Autodesk Inventor part; units mm, degrees
ref_plane "YZ Plane" through (0, 0, 0) normal (1, 0, 0) x (0, 1, 0)
ref_plane "XZ Plane" through (0, 0, 0) normal (0, 1, 0) x (-1, 0, 0)
ref_plane "XY Plane" through (0, 0, 0) normal (0, 0, 1) x (1, 0, 0)
sketch "Sketch1" plane through (0, 0, 0) normal (0, 0, 1) x (1, 0, 0)
  arc A0 (1.5, 7.5) -> (-1.3846, 6.9231) centre (0, 7.5) ccw
  arc A1 (-1.3846, -6.9231) -> (1.5, -7.5) centre (0, -7.5) ccw
  arc A2 (-10.3524, -1.1528) -> (-10.356, 1.1198) centre (-12, -0.0191) ccw
  arc A3 (10.1342, 4.2777) -> (-10.6479, 2.7607) centre (0, 0) ccw
  arc A4 (-10.6391, -2.7946) -> (10.134, -4.278) centre (0, 0) ccw
  arc A5 (-10.6479, 2.7607) -> (-10.356, 1.1198) centre (-8.7119, 2.2588) ccw
  arc A6 (-10.3524, -1.1528) -> (-10.6391, -2.7946) centre (-8.7047, -2.2865) ccw
  arc A7 (-1, 5) -> (-1.3846, 6.9231) centre (-6, 5) ccw
  arc A8 (-1.3846, -6.9231) -> (-1, -5) centre (-6, -5) ccw
  line L0 (1.5, 7.5) -> (1.5, 6.5)
  line L1 (1.4995, -6.5) -> (1.4995, -7.5382)
  line L2 (6.4997, -1.5002) -> (8.2915, -1.5002)
  line L3 (6.4998, 1.5) -> (8.2915, 1.4999)
  arc A9 (6.4997, -1.5002) -> (1.4995, -6.5) centre (6.4995, -6.5002) ccw
  arc A10 (1.5, 6.5) -> (6.4998, 1.5) centre (6.5, 6.5) ccw
  arc A11 (10.134, -4.278) -> (8.2915, -1.5002) centre (8.2915, -3.5002) ccw
  arc A12 (8.2915, 1.4999) -> (10.1342, 4.2777) centre (8.2916, 3.4999) ccw
  line L4 (-6, 2) -> (-4, 2)
  line L5 (-4, -2) -> (-6, -2)
  line L6 (-7, -1) -> (-7, 1)
  arc A13 (-6, 2) -> (-7, 1) centre (-6, 1) ccw
  arc A14 (-7, -1) -> (-6, -2) centre (-6, -1) ccw
  line L7 (-1, -5) -> (-1, -5)
  line L8 (-1, 5) -> (-1, 5)
  arc A15 (-4, 2) -> (-1, 5) centre (-4, 5) ccw
  arc A16 (-1, -5) -> (-4, -2) centre (-4, -5) ccw
  point P0 (10.8972, -1.5003)
  point P1 (10.8973, 1.4999)
  point P2 (1.5, 1.5002)
  point P3 (1.4997, -1.5)
  point P4 (-1, -6.382)
  point P5 (-1, 6.382)
  point P6 (-7, 2)
  point P7 (-7, -2)
  point P8 (-4.7429, 0)
  dimension "d5" = 3
  dimension "d6" = 3
  dimension "d7" = 15
  dimension "d18" = 7.5
  dimension "d20" = 4
  dimension "d21" = 12
  dimension "d22" = 2
  dimension "d26" = 5
  dimension "d27" = 5
  dimension "d28" = 2
  dimension "d30" = 4
  dimension "d31" = 1
  dimension "d32" = 3
  dimension "d33" = 7
extrude "Extrusion2" add sketch "Sketch1" along normal blind 3
properties part number "020914 Aft Middle Endcap" material "Polycarbonate, Clear"
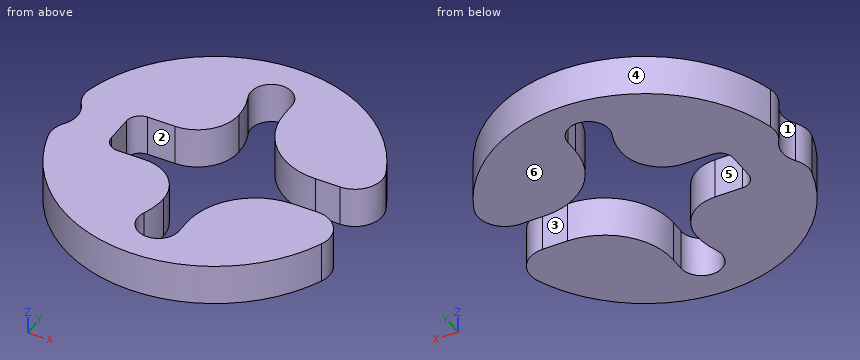
Design review of the part built by this model. Coordinates are the model's own, in mm. Face numbers are marked on the shaded views. A direction names the side the tool comes from. Round coordinates to 2 decimals unless told otherwise and drop trailing zeros. Write each loop counter-clockwise with the first axis right and the second up, starting at its lowest first coordinate (ties: lowest second). Pieces come first, ordered by that corner, then holes. Notation, with made-up numbers: (-30, -22.5) -> (17, -22.5) arc R10 cw to (17, -8.5) -> close; hole circle Ø3 at (-28.5, -38.5). An arc over 180 degrees is marked (long way). Answer in a Markdown table with one row per item.
Q1. Take a section at B-B, the plane y = -4.75. State the section outline as (x, z) points, then the cut area to 3 significant figures.
The answers:
| item | result |
|---|---|
| outline | (-9.92, 0) -> (-1.01, 0) -> (-1.01, 3) -> (-9.92, 3) -> close; (1.82, 0) -> (9.92, 0) -> (9.92, 3) -> (1.82, 3) -> close |
| area | 51.1 mm² |
Q2. Take a section at C-C, the plane z = 2.3. State the section outline as (x, y) points, then the cut area to 3 significant figures.
The answers:
| item | result |
|---|---|
| outline | (-10.65, 2.76) arc R2 ccw to (-10.36, 1.12) arc R2 cw to (-10.35, -1.15) arc R2 ccw to (-10.64, -2.79) arc R11 ccw to (10.13, -4.28) arc R2 ccw to (8.29, -1.5) -> (6.5, -1.5) arc R5 ccw to (1.5, -6.5) -> (1.5, -7.5) arc R1.5 cw (long way) to (-1.38, -6.92) arc R5 ccw to (-1, -5) arc R3 ccw to (-4, -2) -> (-6, -2) arc R1 cw to (-7, -1) -> (-7, 1) arc R1 cw to (-6, 2) -> (-4, 2) arc R3 ccw to (-1, 5) arc R5 ccw to (-1.38, 6.92) arc R1.5 cw (long way) to (1.5, 7.5) -> (1.5, 6.5) arc R5 ccw to (6.5, 1.5) -> (8.29, 1.5) arc R2 ccw to (10.13, 4.28) arc R11 ccw to start |
| area | 262 mm² |
Q3. For the marked faces 1, 2 and 3, list the 3-axis set-ups (+Z, -Z, +X, -X, +Y, -Y) from which the entire face can be reached by the end or side of a thin tool; tool diameter is ignored.
The answers:
| item | result |
|---|---|
| face 1 | +Z, -Z, -X |
| face 2 | +Z, -Z |
| face 3 | +Z, -Z, +X |
Q4. Draft analysis for pull direction Y (two halves, no side actions). For the marked faces 4, 5 and 6, state which applies: +Y half, -Y half, draft (parallel to the pull), parting line (faces both ways), or undercut.
The answers:
| item | result |
|---|---|
| face 4 | +Y half |
| face 5 | undercut |
| face 6 | draft |
Q5. Take a section at A-A, the plane x = -2.5. State the section outline as (y, z) points.
The answers:
| item | result |
|---|---|
| outline | (-10.71, 0) -> (-2.4, 0) -> (-2.4, 3) -> (-10.71, 3) -> close; (2.4, 0) -> (10.71, 0) -> (10.71, 3) -> (2.4, 3) -> close |
Q6. Clearance check with flat-ended pins moving along their axes: pin 1 Ø1 at (y, z) = (0, 1.5) entering from +X; pin 2 Ø1.5 at (y, z) = (-5, 0.5) entering from +X; pin 3 Ø0.9 at (x, z) = (7.5, 1.5) entering from -Y; pin 4 Ø2.5 at (x, y) = (0, -7.5) entering from +Z. State where each tip first meets the part, or that it passes through.
The answers:
| item | result |
|---|---|
| pin 1 | x = -7 |
| pin 2 | x = 10.15 |
| pin 3 | y = -8.44 |
| pin 4 | through |
Q7. To check wall thickness, follow L1, parallel to X at y = 7, z = 0.25; L2, parallel to X at y = 7.75, z = 1.5; L3, parallel to Y at x = 4.5, z = 0.5. State the ranges of each line that lie inside material, in increasing order. Write a range as [from, to].
The answers:
| item | result |
|---|---|
| L1 | [-8.49, -1.41], [1.5, 8.49] |
| L2 | [-7.81, -1.48], [1.48, 7.81] |
| L3 | [-10.04, -1.92], [1.92, 10.04] |
